Source: CAD feature listing. Evaluate the final solid. Frame: model axes, mm. Face numbers are marked on the shaded views. A direction names the side the tool comes from. Coordinates: 2 decimals unless noted, no trailing zeros. Write each loop counter-clockwise with the first axis right and the second up, starting at its lowest first coordinate (ties: lowest second). Pieces come first, ordered by that corner, then holes. Notation, with made-up numbers: (74, 30) - (94, 30) arc R14 ccw to (94, 50) - close; hole circle Ø3 at (20, -15). An arc over 180 degrees is marked (long way). One line per question, with ' | ' between items.
Autodesk Inventor part; units mm, degrees
ref_plane "Work Plane7" through (-10, 4, 4) normal (0, 0.7071, -0.7071) x (-1, 0, 0)
ref_plane "YZ Plane" through (0, 0, 0) normal (1, 0, 0) x (0, 1, 0)
ref_plane "XZ Plane" through (0, 0, 0) normal (0, 1, 0) x (-1, 0, 0)
sketch "_____1" plane through (0, 0, 0) normal (1, 0, 0) x (0, 0, -1)
  line L0 (-30, 2.6786) -> (-30, 0)
  line L1 (-30, 0) -> (0, 0)
  line L2 (0, 0) -> (0, 30)
  line L3 (0, 30) -> (-2.6786, 30)
  arc A0 (-2.6786, 30) -> (-3.815, 29.5293) centre (-2.6786, 28.3929) ccw
  line L4 (-3.815, 29.5293) -> (-29.5293, 3.815)
  arc A1 (-29.5293, 3.815) -> (-30, 2.6786) centre (-28.3929, 2.6786) ccw
  dimension "d42" = 30
extrude "Extrusion1" add sketch "_____1" along normal mid plane 20
sketch "_____2" plane through (0, 0, 0) normal (1, 0, 0) x (0, 0, -1)
  line L0 (-32, 32) -> (-32, 4)
  line L1 (-32, 4) -> (-6, 4)
  arc A0 (-6, 4) -> (-4, 6) centre (-6, 6) ccw
  line L2 (-4, 6) -> (-4, 32)
  line L3 (-4, 32) -> (-32, 32)
extrude "Extrusion2" cut sketch "_____2" along normal mid plane 30
sketch "_____9" plane through (0, 0, 0) normal (1, 0, 0) x (0, 0, -1)
  line L0 (0, 5) -> (0, 1.8718)
  line L1 (0, 1.8718) -> (1.592, 2.2984)
  arc A0 (1.592, 2.2984) -> (2, 2.7898) centre (1.5, 2.7898) ccw
  line L2 (2, 2.7898) -> (2, 4.7898)
  arc A1 (2, 4.7898) -> (1.9797, 4.9309) centre (1.5, 4.7898) ccw
  line L3 (1.9797, 4.9309) -> (0, 5)
  line L4 (-30, 0) -> (0, 0)
  line L5 (0, 0) -> (0, 30)
  dimension "d34" = 0.5
  dimension "d35" = 0.5
  dimension "d36" = 15
  dimension "d37" = 2
  dimension "d38" = 2
  dimension "d40" = 2
  dimension "d41" = 5
extrude "Extrusion3" add sketch "_____9" along normal mid plane 8
sketch "_____10" plane through (0, 0, 0) normal (1, 0, 0) x (0, 0, -1)
  line L0 (-5.2401, 0) -> (-5.1188, -2.524)
  arc A0 (-5.1188, -2.524) -> (-4.6194, -3) centre (-4.6194, -2.5) ccw
  line L1 (-4.6194, -3) -> (-3.0897, -3)
  arc A1 (-3.0897, -3) -> (-2.6413, -2.7213) centre (-3.0897, -2.5) ccw
  line L2 (-2.6413, -2.7213) -> (-1.298, 0)
  line L3 (-1.298, 0) -> (-5.2401, 0)
  line L4 (0, 0) -> (-30, 0)
  line L5 (0, 30) -> (0, 0)
  dimension "d26" = 0.5
  dimension "d27" = 0.5
  dimension "d28" = 3
  dimension "d29" = 2.749
extrude "Extrusion4" add sketch "_____10" along normal mid plane 8
sketch "_____3" plane through (0, 0, 0) normal (0, 1, 0) x (1, 0, 0)
  arc A0 (-3.2, -12) -> (3.2, -12) centre (0, -12) ccw
  line L0 (3.2, -12) -> (3.2, -6)
  line L1 (3.2, -6) -> (-3.2, -6)
  line L2 (-3.2, -6) -> (-3.2, -12)
  line L3 (-10, 0) -> (10, 0)
  line L4 (0, -6) -> (0, 0) construction
  point P0 (-3.2, -9)
  point P1 (3.2, -9)
  dimension "d23" = 3.2
  dimension "d24" = 6
  dimension "d25" = 6
extrude "Extrusion5" cut sketch "_____3" along normal blind 4
ref_plane "Work Plane7" through (-10, 4, 4) normal (0, 0.7071, -0.7071) x (-1, 0, 0)
mirror "Mirror1" about plane through (-10, 4, 4) normal (0, 0.7071, -0.7071) of "Extrusion5"
properties part number "HBLFSR5_b" material "Acetal Resin, Black"
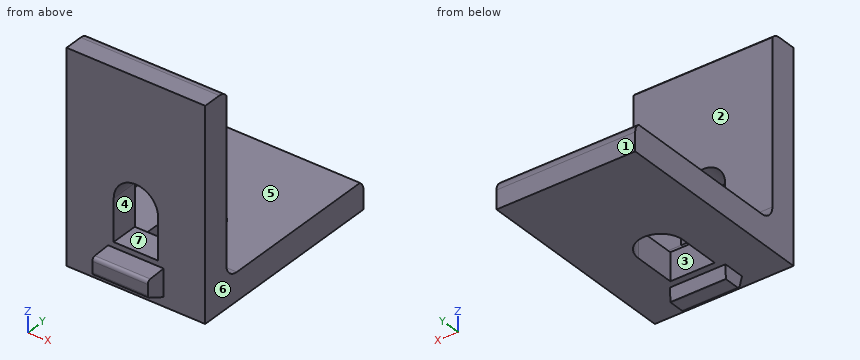
Item 1: Cut plane C-C on z = 13. Return loops of the section in (x, y).
Check sheet entries:
outline: (-10, 0) - (-3.04, 0) - (-3.04, 4) - (-10, 4) - close; (3.04, 0) - (10, 0) - (10, 4) - (3.04, 4) - close
Item 2: Cut plane B-B on x = 0. State how many separate pieces and enclosed holes the cut face has, and give its area (3 significant figures).
Check sheet entries:
separate pieces: 3 | enclosed holes: 0 | area: 166 mm²
Item 3: Cut plane D-D on x = -5. Return loops of the section in (y, z) (3 decimals), and give its area (3 significant figures).
Check sheet entries:
outline: (0, 0) - (30, 0) - (30, 2.679) arc R1.607 ccw to (29.529, 3.815) - (29.344, 4) - (6, 4) arc R2 cw to (4, 6) - (4, 29.344) - (3.815, 29.529) arc R1.607 ccw to (2.679, 30) - (0, 30) - close | area: 224 mm²
Item 4: Mould query, pull axis Z, two halves, no side actions, for the marked faces 4, 5, 6 and 7. Classes: pulls with the +Z half, pulls with the -Z half, needs draft (parallel to the pull), parting line crosses it, or undercut.
Check sheet entries:
face 4: undercut | face 5: pulls with the +Z half | face 6: needs draft | face 7: undercut
Item 5: Cut plane A-A on y = 6.5. Return loops of the section in (x, z), and give its area (3 significant figures).
Check sheet entries:
outline: (-10, 0) - (-3.2, 0) - (-3.2, 4) - (-10, 4) - close; (3.2, 0) - (10, 0) - (10, 4) - (3.2, 4) - close | area: 54.4 mm²
Item 6: Ray query, line 1 along Y through (x, z) = (1.5, 19); line 2 along Y through (x, z) = (5.5, 2). Return the intervals inside material, ascending. Write a range as [from, to].
Check sheet entries:
line 1: [0, 4] | line 2: [0, 30]
Item 7: Pin query (flat end, axial travel): pin 1 Ø2 at (x, y) = (-7.5, 14) entering from +Z; pin 2 Ø0.6 at (y, z) = (3.5, -1.5) entering from +X; pin 3 Ø6 at (x, z) = (3, 20.5) entering from -Y; pin 4 Ø1 at (y, z) = (5, 6.5) entering from -X. Return the tip coordinate at first contact, or that it passes through.
Check sheet entries:
pin 1: z = 4 | pin 2: x = 4 | pin 3: y = 0 | pin 4: through
Item 8: Access query for the marked faces 1, 2 and 3. Directions: +Z, -Z, +X, -X, +Y, -Y. A direction counts if a zero-diameter tool reaches every point of the face in a straight line with its end or side. Return the directions, or none.
Check sheet entries:
face 1: +Z, -Z, +X, -X, +Y | face 2: +Z, +X, -X, +Y | face 3: +Z, -Z
